```python
from build123d import *

# Parameters (mm, degrees)
SKETCH_4_W          = 5
SKETCH_4_H          = 10
EXTRUDE_2_DEPTH     = 4.5
SKETCH_5_W          = 4.5
SKETCH_5_H          = 7
EXTRUDE_3_DEPTH     = 1
SKETCH_6_W          = 4.5
SKETCH_6_H          = 7
EXTRUDE_4_DEPTH     = 1
SKETCH_7_R          = 2.25
EXTRUDE_5_DEPTH     = 0.5
SKETCH_8_R          = 0.25
CUT_EXTRUDE_1_DEPTH = 0.5
CUT_EXTRUDE_START   = -0.5
SKETCH_9_R          = 0.25
CUT_EXTRUDE_2_DEPTH = 0.5
SCALE_1_SCALE       = 3.181818182
SCALE_2_SCALE       = 2.454545455
SCALE_3_SCALE       = 0.771428571
SCALE_4_SCALE       = 0.407393437
SKETCH_10_W         = 14.212580929
SKETCH_10_H         = 3.204768758
CUT_EXTRUDE_3_DEPTH = 20.209197968


with BuildPart() as part:
    # 草图4 → 凸台-拉伸2 (new body)
    with BuildSketch(Plane.XY):
        Rectangle(SKETCH_4_W, SKETCH_4_H)
    extrude(amount=EXTRUDE_2_DEPTH)

    # 草图5 → 凸台-拉伸3 (add)
    with BuildSketch(Plane(origin=(2.5, 0, 0), x_dir=(0, 0, -1), z_dir=(1, 0, 0))):
        with Locations((-2.25, 0)):
            Rectangle(SKETCH_5_W, SKETCH_5_H)
    extrude(amount=EXTRUDE_3_DEPTH)

    # 草图6 → 凸台-拉伸4 (add)
    with BuildSketch(Plane.ZY.offset(2.5)):
        with Locations((2.25, 0)):
            Rectangle(SKETCH_6_W, SKETCH_6_H)
    extrude(amount=EXTRUDE_4_DEPTH)

    # 草图7 → 凸台-拉伸5 (add)
    with BuildSketch(Plane(origin=(3.5, 0, 0), x_dir=(0, 0, -1), z_dir=(1, 0, 0))):
        with Locations((-2.25, 0)):
            Circle(SKETCH_7_R)
    extrude_5 = extrude(amount=EXTRUDE_5_DEPTH)

    # 镜向1: 凸台-拉伸5 across plane
    add(extrude_5.mirror(Plane(origin=(0, 0, 0), x_dir=(0, 0, 1), z_dir=(1, 0, 0))))

    # 草图8 → 切除-拉伸1 (cut)
    with BuildSketch(Plane(origin=(4, 0, 0), x_dir=(0, 0, -1), z_dir=(1, 0, 0))):
        with Locations((-2.25, 0)):
            Circle(SKETCH_8_R)
    extrude(amount=-CUT_EXTRUDE_1_DEPTH, mode=Mode.SUBTRACT)

    # 草图9 → 切除-拉伸2 (cut)
    with BuildSketch(Plane.ZY.offset(4).offset(CUT_EXTRUDE_START)):
        with Locations(Location((2.25, 0, 0), (0, 0, 180))):
            Circle(SKETCH_9_R)
    extrude(amount=CUT_EXTRUDE_2_DEPTH, mode=Mode.SUBTRACT)


with BuildPart() as part_1:
    # 缩放比例1: scaled about (0, 0, 2.25)
    add(part.part.scale(SCALE_1_SCALE).moved(Location((0, 0, -4.909090909))))


with BuildPart() as part_2:
    # 缩放比例2: scaled about (0, 0, 2.25)
    add(part_1.part.scale(SCALE_2_SCALE).moved(Location((0, 0, -3.272727273))))


with BuildPart() as part_3:
    # 缩放比例3: scaled about (0, 0, 2.25)
    add(part_2.part.scale(SCALE_3_SCALE).moved(Location((0, 0, 0.514285714))))


with BuildPart() as part_4:
    # 缩放比例4: scaled about (0, 0, 2.25)
    add(part_3.part.scale(SCALE_4_SCALE).moved(Location((0, 0, 1.333364768))))

    # 草图10 → 切除-拉伸3 (cut, through all)
    with BuildSketch(Plane(origin=(0, 0, -3.272537886), x_dir=(-1, 0, 0), z_dir=(0, 0, -1))):
        with Locations((0.970137257, 13.104690793)):
            Rectangle(SKETCH_10_W, SKETCH_10_H)
    extrude(amount=-CUT_EXTRUDE_3_DEPTH, mode=Mode.SUBTRACT)


solid = part_4.part
```
Check sheet for the modelled part. Datum: model origin and axes. Units: mm. A direction names the side the tool comes from. Coordinates: 2 decimals unless noted, no trailing zeros. Write each loop counter-clockwise with the first axis right and the second up, starting at its lowest first coordinate (ties: lowest second). Pieces come first, ordered by that corner, then holes. Notation, with made-up numbers: (9, 1) - (53, 1) arc R33 cw to (53, 40) - close; hole circle Ø10 at (8, 64). An arc over 180 degrees is marked (long way). One line per question, with ' | ' between items.
Item 1: Thickness scan on line 1 (Y direction, x = -9.1, z = 2.25); line 2 (Y direction, x = -7, z = 0.5). Record the ranges inside material, lowest first. Write a range as [from, to].
Determined:
line 1: y = [-5.52, -0.61], [0.61, 5.52] | line 2: y = [-8.59, 8.59]
Item 2: Sectioned sample at B-B on y = 10.25. Record the boundary of the cut face in (x, z).
Determined:
outline: (-6.14, -3.27) - (6.14, -3.27) - (6.14, 7.77) - (-6.14, 7.77) - close
Item 3: Sectioned sample at A-A on z = 2.25. Record the boundary of the cut face in (x, y), plus the area to 3 significant figures.
Determined:
outline: (-9.82, -5.52) - (-8.59, -5.52) - (-8.59, -8.59) - (-6.14, -8.59) - (-6.14, -12.27) - (6.14, -12.27) - (6.14, -8.59) - (8.59, -8.59) - (8.59, -5.52) - (9.82, -5.52) - (9.82, -0.61) - (8.59, -0.61) - (8.59, 0.61) - (9.82, 0.61) - (9.82, 5.52) - (8.59, 5.52) - (8.59, 8.59) - (6.14, 8.59) - (6.14, 11.5) - (-6.14, 11.5) - (-6.14, 8.59) - (-8.59, 8.59) - (-8.59, 5.52) - (-9.82, 5.52) - (-9.82, 0.61) - (-8.59, 0.61) - (-8.59, -0.61) - (-9.82, -0.61) - close | area: 400 mm2
Item 4: Access from +Z, -Z, +X, -X, +Y, -Y to the whole of each face (thin tool, end or side, straight path). Record for faces 5 (the face through (-9.196, 0.243, 7.767)), 6 (the face through (9.196, 0.243, 7.767)), 7 (the face through (-7, 8.591, 2)), 8 (the face through (-6.136, -10, 2)), 9 (the face through (6.136, 10, 2)).
Determined:
face 5: -X | face 6: +X | face 7: +Z, -Z, -X, +Y | face 8: +Z, -Z, -X, -Y | face 9: +Z, -Z, +X, +Y
Item 5: Mould release check, pull along Z, two halves, no side actions. Record for faces 1 (the face through (9.213, 0.184, 1.665)), 2 (the face through (-8.591, 0, 2)), 3 (the face through (7, 8.591, 2)), 4 (the face through (0, 0, 7.773)): pulls with the +Z half, pulls with the -Z half, needs draft (parallel to the pull), parting line crosses it, or undercut.
Determined:
face 1: undercut | face 2: undercut | face 3: needs draft | face 4: pulls with the +Z half
Item 6: Sectioned sample at C-C on x = 8.25. Record the boundary of the cut face in (y, z), plus the area to 3 significant figures.
Determined:
outline: (-8.59, -3.27) - (8.59, -3.27) - (8.59, 7.77) - (-8.59, 7.77) - close | area: 190 mm2
Item 7: Gauge pin test, flat ends, axial feed: P1, Ø6, axis at y = -9, z = 3, coming from the -X side; P2, Ø0.9, axis at y = 9.5, z = 0, coming from the -X side; P3, Ø4, axis at y = -11, z = 3.5, coming from the +X side. Record the tip position at first contact, or that the pin passes through.
Determined:
P1: stops at x = -8.59 | P2: stops at x = -6.14 | P3: stops at x = 6.14
Item 8: Sectioned sample at D-D on z = 6. Record the boundary of the cut face in (x, y), plus the area to 3 significant figures.
Determined:
outline: (-9.82, -4.05) - (-8.59, -4.05) - (-8.59, -8.59) - (-6.14, -8.59) - (-6.14, -12.27) - (6.14, -12.27) - (6.14, -8.59) - (8.59, -8.59) - (8.59, -4.05) - (9.82, -4.05) - (9.82, 4.05) - (8.59, 4.05) - (8.59, 8.59) - (6.14, 8.59) - (6.14, 11.5) - (-6.14, 11.5) - (-6.14, 8.59) - (-8.59, 8.59) - (-8.59, 4.05) - (-9.82, 4.05) - close | area: 396 mm2
